from build123d import *

# Parameters (mm, degrees)
EXTRUDE_1_DEPTH     = 15
SKETCH_2_R          = 3
EXTRUDE_2_DEPTH     = 8
SKETCH_3_R          = 3
CUT_EXTRUDE_1_DEPTH = 14
CHAMFER_1_SIZE      = 0.1
CHAMFER_1_SIZE2     = 0.057735027
CHAMFER_2_SIZE      = 0.1


with BuildPart() as part:
    # 草图1 → 凸台-拉伸1 (new body)
    with BuildSketch(Plane(origin=(0, 0, 0), x_dir=(1, 0, 0), z_dir=(0, 1, 0))):
        Polygon((2.309401077, 4), (-2.309401077, 4), (-4.618802154, 0), (-2.309401077, -4), (2.309401077, -4), (4.618802154, 0), align=None)
    extrude(amount=EXTRUDE_1_DEPTH)

    # 草图2 → 凸台-拉伸2 (add)
    with BuildSketch(Plane.XZ):
        with Locations(Location((0, 0, 0), (0, 0, 270))):
            Circle(SKETCH_2_R)
    extrude(amount=EXTRUDE_2_DEPTH)

    # 草图3 → 切除-拉伸1 (cut)
    with BuildSketch(Plane(origin=(0, 15, 0), x_dir=(1, 0, 0), z_dir=(0, 1, 0))):
        with Locations(Location((0, 0, 0), (0, 0, 90))):
            Circle(SKETCH_3_R)
    extrude(amount=-CUT_EXTRUDE_1_DEPTH, mode=Mode.SUBTRACT)

    # 草图4 → 切除-旋转1 (revolve, cut)
    with BuildSketch(Plane.XY, mode=Mode.PRIVATE) as cut_revolve_1_sk:
        Polygon((-4.618802154, 0.235852712), (-4.618802154, 0), (-3.970802154, 0), align=None)
        Polygon((-4.618802154, 15), (-4.618802154, 14.764147288), (-3.970802154, 15), align=None)
    revolve(cut_revolve_1_sk.sketch.rotate(Axis((0, -9.15, 0), (0, 1, 0)), 60.000004036), axis=Axis((0, -9.15, 0), (0, 1, 0)), mode=Mode.SUBTRACT)

    # 倒角1
    chamfer_1_edges = [part.edges().sort_by_distance(p)[0] for p in [
        (0, -8, 3),
    ]]
    chamfer_1_side = [part.faces().sort_by_distance(p)[0] for p in [
        (0, -4, 3),
    ]]
    chamfer(chamfer_1_edges, length=CHAMFER_1_SIZE, length2=CHAMFER_1_SIZE2, reference=chamfer_1_side[0])

    # 倒角2
    chamfer_2_edges = [part.edges().sort_by_distance(p)[0] for p in [
        (0, 15, 3),
    ]]
    chamfer(chamfer_2_edges, length=CHAMFER_2_SIZE)


solid = part.part
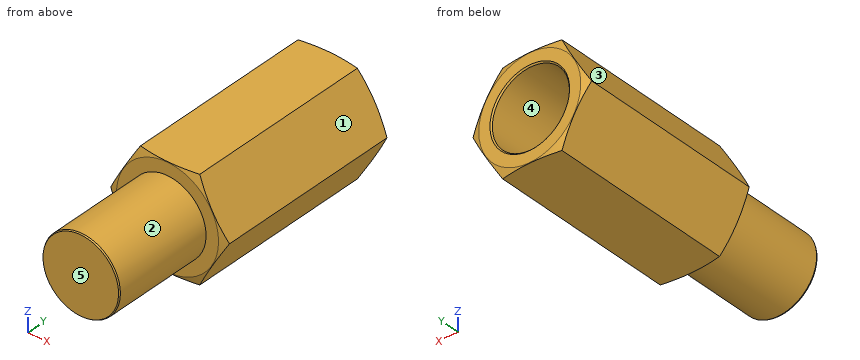
Could you check a few things on this model? Use its own coordinates, in mm. Face numbers are marked on the shaded views. A direction names the side the tool comes from. Coordinates: 2 decimals unless noted, no trailing zeros. Order: outer loops, then holes, each group sorted by start corner. A loop starts at its lowest first (then second) coordinate and runs counter-clockwise, first axis right, second up.
Q1. Suppose I cut it at C-C on y = -2. Please give me the cut outline in (x, z), and give its area (3 significant figures).
Q2. Please list where these lines run through material, in increasing order: L1, parallel to Y at x = 1.5, z = 3; L2, parallel to Y at x = 1, z = 1.75; L3, parallel to X at y = 9.75, z = -2.
Q3. Which directions (+Z, -Z, +X, -X, +Y, -Y) give clear straight access to the entire face, cutting with the end or side of a thin tool? Please do the marked faces 1 and 2.
Q4. Will these pins go through, and if not, where does the flat tip stop? pin 1 (1.5 mm diameter, centred on y = 7, z = 0.5, fed in from -X); pin 2 (1 mm diameter, centred on x = 0.5, z = 0.5, fed in from +Y); pin 3 (2 mm diameter, centred on y = 12.5, z = -2, fed in from +X).
Q5. Thinking about a two-plate mould opening in X: for the marked faces 3, 4 and 5, which applies, released by +X, released by -X, zero draft, split by the parting line, or undercut?
Q6. Suppose I cut it at B-B on y = 4.75. Please give me the cut outline in (x, z).
Answer:
1. outline: circle Ø6 at (0, 0)
1. area: 28.3 mm2
2. L1: y = 0 to 15
2. L2: y = -8 to 1
2. L3: x = -3.46 to -2.24, 2.24 to 3.46
3. face 1: +Z, +X, +Y, -Y
3. face 2: -Y
4. pin 1: stops at x = -4.62
4. pin 2: stops at y = 1
4. pin 3: stops at x = 4.04
5. face 3: released by -X
5. face 4: undercut
5. face 5: zero draft
6. outline: (-4.62, 0) - (-2.31, -4) - (2.31, -4) - (4.62, 0) - (2.31, 4) - (-2.31, 4) - close; hole circle Ø6 at (0, 0)
